from build123d import *
from build123d import SkipClean  # not in build123d's __all__

# Parameters (mm, degrees)
F0_R     = 32.5
F0_R_2   = 4
F0_R_3   = 2.25
F1_DEPTH = 3
F2_START = 3
F2_DEPTH = 13
F3_START = 3
F3_DEPTH = 13
F5_START = 3
F5_DEPTH = 4
F6_START = 7
F6_DEPTH = 10


# Not quite as in the source:
# - a fillet or chamfer that OpenCascade refuses, or shapes differently, is made with other operations: its cross-section is extruded or revolved along the edge and cut away or added


with BuildPart() as f1:
    # F0 (on Top) → F1 (new body)
    with BuildSketch(Plane.XY):
        Circle(F0_R)
        with Locations((-25, -5.0249378106)):
            Circle(F0_R_2, mode=Mode.SUBTRACT)
        with BuildLine():
            ThreePointArc((25, -16.5831239518), (0, -30), (-25, -16.5831239518))
            Line((-25, -16.5831239518), (-23.2643659014, -15.5810551377))
            Line((-23.2643659014, -15.5810551377), (23.2643659014, -15.5810551377))
            Line((23.2643659014, -15.5810551377), (25, -16.5831239518))
        make_face(mode=Mode.SUBTRACT)
        with Locations((25, -5.0249378106)):
            Circle(F0_R_2, mode=Mode.SUBTRACT)
        with BuildLine():
            ThreePointArc((1.375, 20.2562448003), (3.2787192622, 18.7912878475), (4, 16.5))
            ThreePointArc((4, 16.5), (3.2787192622, 14.2087121525), (1.375, 12.7437551997))
            ThreePointArc((1.375, 12.7437551997), (0, 12.5), (-1.375, 12.7437551997))
            ThreePointArc((-1.375, 12.7437551997), (-4, 16.5), (-1.375, 20.2562448003))
            ThreePointArc((-1.375, 20.2562448003), (0, 20.5), (1.375, 20.2562448003))
        make_face(mode=Mode.SUBTRACT)
        with BuildLine():
            Line((23.2643659014, -15.5810551377), (-23.2643659014, -15.5810551377))
            ThreePointArc((-23.2643659014, -15.5810551377), (0, -28), (23.2643659014, -15.5810551377))
        make_face()
        with BuildLine():
            Line((-23.2643659014, -15.5810551377), (-25, -16.5831239518))
            ThreePointArc((-25, -16.5831239518), (0, -30), (25, -16.5831239518))
            Line((25, -16.5831239518), (23.2643659014, -15.5810551377))
            ThreePointArc((23.2643659014, -15.5810551377), (0, -28), (-23.2643659014, -15.5810551377))
        make_face()
        with Locations((25, -5.0249378106)):
            Circle(F0_R_2)
        with Locations((25, -5.0249378106)):
            Circle(F0_R_3, mode=Mode.SUBTRACT)
        with Locations((-25, -5.0249378106)):
            Circle(F0_R_2)
        with Locations((-25, -5.0249378106)):
            Circle(F0_R_3, mode=Mode.SUBTRACT)
        with BuildLine():
            Line((1.375, 12.7437551997), (1.375, 20.2562448003))
            ThreePointArc((1.375, 20.2562448003), (0, 20.5), (-1.375, 20.2562448003))
            Line((-1.375, 20.2562448003), (-1.375, 12.7437551997))
            ThreePointArc((-1.375, 12.7437551997), (0, 12.5), (1.375, 12.7437551997))
        make_face()
        with Locations((25, -5.0249378106)):
            Circle(F0_R_3)
        with Locations((-25, -5.0249378106)):
            Circle(F0_R_3)
        with BuildLine():
            ThreePointArc((1.375, 12.7437551997), (3.2787192622, 14.2087121525), (4, 16.5))
            ThreePointArc((4, 16.5), (3.2787192622, 18.7912878475), (1.375, 20.2562448003))
            Line((1.375, 20.2562448003), (1.375, 12.7437551997))
        make_face()
        with BuildLine():
            Line((-1.375, 12.7437551997), (-1.375, 20.2562448003))
            ThreePointArc((-1.375, 20.2562448003), (-4, 16.5), (-1.375, 12.7437551997))
        make_face()
    extrude(amount=F1_DEPTH)

    # F0 (on Top) → F2 (join)
    with BuildSketch(Plane.XY.offset(F2_START)):
        with BuildLine():
            Line((-23.2643659014, -15.5810551377), (-25, -16.5831239518))
            ThreePointArc((-25, -16.5831239518), (0, -30), (25, -16.5831239518))
            Line((25, -16.5831239518), (23.2643659014, -15.5810551377))
            ThreePointArc((23.2643659014, -15.5810551377), (0, -28), (-23.2643659014, -15.5810551377))
        make_face()
    extrude(amount=F2_DEPTH)

    # F0 (on Top) → F3 (join)
    with BuildSketch(Plane.XY.offset(F3_START)):
        with Locations((-25, -5.0249378106)):
            Circle(F0_R_2)
        with Locations((-25, -5.0249378106)):
            Circle(F0_R_3, mode=Mode.SUBTRACT)
        with Locations((25, -5.0249378106)):
            Circle(F0_R_2)
        with Locations((25, -5.0249378106)):
            Circle(F0_R_3, mode=Mode.SUBTRACT)
    extrude(amount=F3_DEPTH)

    # F4: chamfer of 2 x 1.4004150764 on 2 edges, made by hand

    # F4_s1 → F4_t2 (revolve, cut)
    with BuildSketch(Plane.XZ.offset(5.0249378106)):
        Polygon((-21, 14.5995849236), (-23, 16), (-21, 16), align=None)
    revolve(axis=Axis((-25, -5.0249378106, 16), (0, 0, 1)), mode=Mode.SUBTRACT)

    # F4_s3 → F4_t4 (revolve, cut)
    with BuildSketch(Plane.XZ.offset(5.0249378106)):
        Polygon((29, 14.5995849236), (27, 16), (29, 16), align=None)
    revolve(axis=Axis((25, -5.0249378106, 16), (0, 0, 1)), mode=Mode.SUBTRACT)

    # F0 (on Top) → F5 (join)
    with BuildSketch(Plane.XY.offset(F5_START)):
        with BuildLine():
            ThreePointArc((1.375, 12.7437551997), (3.2787192622, 14.2087121525), (4, 16.5))
            ThreePointArc((4, 16.5), (3.2787192622, 18.7912878475), (1.375, 20.2562448003))
            Line((1.375, 20.2562448003), (1.375, 12.7437551997))
        make_face()
        with BuildLine():
            Line((-1.375, 12.7437551997), (-1.375, 20.2562448003))
            ThreePointArc((-1.375, 20.2562448003), (-4, 16.5), (-1.375, 12.7437551997))
        make_face()
        with BuildLine():
            Line((1.375, 12.7437551997), (1.375, 20.2562448003))
            ThreePointArc((1.375, 20.2562448003), (0, 20.5), (-1.375, 20.2562448003))
            Line((-1.375, 20.2562448003), (-1.375, 12.7437551997))
            ThreePointArc((-1.375, 12.7437551997), (0, 12.5), (1.375, 12.7437551997))
        make_face()
    extrude(amount=F5_DEPTH)

    # F0 (on Top) → F6 (join)
    with BuildSketch(Plane.XY.offset(F6_START)):
        with BuildLine():
            Line((-1.375, 12.7437551997), (-1.375, 20.2562448003))
            ThreePointArc((-1.375, 20.2562448003), (-4, 16.5), (-1.375, 12.7437551997))
        make_face()
        with BuildLine():
            ThreePointArc((1.375, 12.7437551997), (3.2787192622, 14.2087121525), (4, 16.5))
            ThreePointArc((4, 16.5), (3.2787192622, 18.7912878475), (1.375, 20.2562448003))
            Line((1.375, 20.2562448003), (1.375, 12.7437551997))
        make_face()
    with SkipClean():  # cleaning this boolean's faces spoils the solid; the shape is the same uncleaned
        extrude(amount=F6_DEPTH)


solid = f1.part
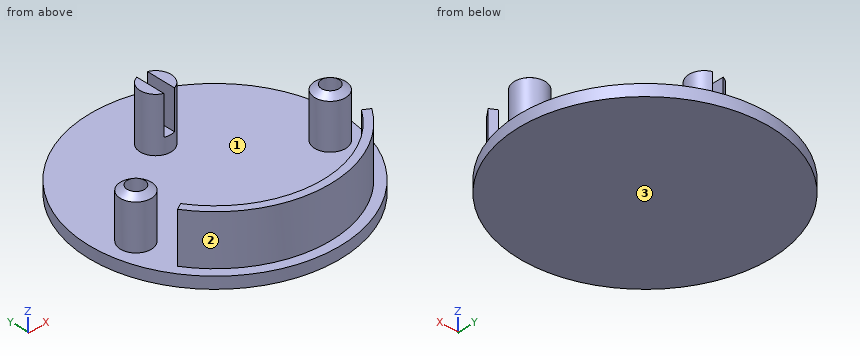
Verification items for the finished model (mm, model axes). Face numbers are marked on the shaded views. Coordinates: 2 decimals unless noted, no trailing zeros. Loops run counter-clockwise (first coordinate to the right, second up) from the corner with the lowest first, then second, coordinate; pieces in that order, holes last. Notation, with made-up numbers: (3, 22) -> (9, 22) arc R21 ccw to (9, 47) -> close; hole circle Ø5 at (47.5, -11.5). An arc over 180 degrees is marked (long way). Answer as CSV lines item,"result".
1) Depth check by flat-ended pin: pin 1 (6 mm diameter, centred on y = 17.5, z = 11, fed in from -X); pin 2 (10 mm diameter, centred on x = 24.5, z = 13.5, fed in from +Y); pin 3 (6 mm diameter, centred on x = -25, y = -5.02, fed in from +Z). Enter the tip coordinate at first touch or a pass-through.
Found:
pin 1,"stops at x = -4"
pin 2,"stops at y = -1.02"
pin 3,"stops at z = 15.82"
2) Release check for a two-part mould opening along Y. For the marked faces 1, 2 and 3 record: +Y half, -Y half, draft (parallel to the pull), parting line (faces both ways), or undercut.
Found:
face 1,"undercut"
face 2,"-Y half"
face 3,"draft"
3) Thickness scan on L1, parallel to X at y = -3, z = 14.25; L2, parallel to X at y = -4, z = 5.25; L3, parallel to Z at x = 6, y = 21. Record the ranges inside material, lowest first. Write a range as from..to.
Found:
L1,"x = -28.45..-25.98, -24.02..-21.55, 21.55..24.02, 25.98..28.45"
L2,"x = -28.87..-27, -23..-21.13, 21.13..23, 27..28.87"
L3,"z = 0..3"
4) Cross-section at D-D, the plane y = 14. Record the cut outline in (x, z) (1 decimal).
Found:
outline,"(-29.3, 0) -> (29.3, 0) -> (29.3, 3) -> (3.1, 3) -> (3.1, 17) -> (1.4, 17) -> (1.4, 7) -> (-1.4, 7) -> (-1.4, 17) -> (-3.1, 17) -> (-3.1, 3) -> (-29.3, 3) -> close"
5) Cross-section at C-C, the plane y = 0. Record the cut outline in (x, z), then the cut area to 3 significant figures.
Found:
outline,"(-32.5, 0) -> (32.5, 0) -> (32.5, 3) -> (-32.5, 3) -> close"
area,"195 mm2"
6) Cross-section at A-A, the plane z = 8.5. Record the cut outline in (x, y) (3 decimals), then the cut area to 3 significant figures.
Found:
outline,"circle Ø8 at (-25, -5.025); (-25, -16.583) arc R30 ccw to (25, -16.583) -> (23.264, -15.581) arc R28 cw to (-23.264, -15.581) -> close; (-1.375, 12.744) -> (-1.375, 20.256) arc R4 ccw to start; (1.375, 12.744) arc R4 ccw to (1.375, 20.256) -> close; circle Ø8 at (25, -5.025); hole circle Ø4.5 at (-25, -5.025); hole circle Ø4.5 at (25, -5.025)"
area,"211 mm2"
7) Cross-section at B-B, the plane x = -5. Record the cut outline in (y, z), then the cut area to 3 significant figures.
Found:
outline,"(-32.11, 0) -> (32.11, 0) -> (32.11, 3) -> (-27.55, 3) -> (-27.55, 16) -> (-29.58, 16) -> (-29.58, 3) -> (-32.11, 3) -> close"
area,"219 mm2"
